Geometry check sheet. Reference: the model listing, model coordinates, mm. Face numbers are marked on the shaded views. A direction names the side the tool comes from. Give positions to 0.01 mm unless a question says otherwise; leave off trailing zeros. Loops run counter-clockwise (first coordinate to the right, second up) from the corner with the lowest first, then second, coordinate; pieces in that order, holes last.
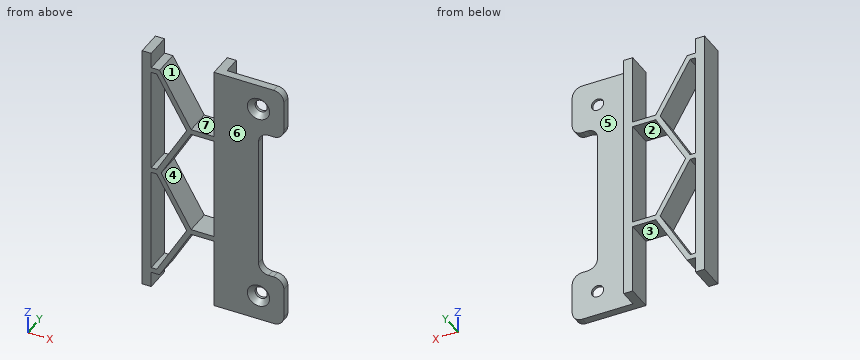
```python
from build123d import *

# Parameters (mm, degrees)
BOSS_EXTRUDE1_DEPTH                            = 5
BOSS_EXTRUDE3_DEPTH                            = 1.5
FILLET1_R                                      = 2
CSK_FOR_M2_FLAT_HEAD_MACHINE_SCREW1_AT_2_COUNT = 2
CSK_FOR_M2_FLAT_HEAD_MACHINE_SCREW1_AT_2_PITCH = 40


with BuildPart() as part:
    # Sketch1 → Boss-Extrude1 (new body)
    with BuildSketch(Plane(origin=(0, 0, 0), x_dir=(1, 0, 0), z_dir=(0, 1, 0))):
        Polygon((-14.18, 46.928571429), (-14.18, 50), (-15.96, 50), (-15.96, 0), (-14.18, 0), (-14.18, 3.071428571), (-12.513875906, 3.071428571), (-6.313875906, 13.785714286), (-1.78, 13.785714286), (-1.78, 0), (0, 0), (0, 50), (-1.78, 50), (-1.78, 36.214285714), (-6.313875906, 36.214285714), (-12.513875906, 46.928571429), align=None)
        Polygon((-14.18, 4.071428571), (-14.18, 24.5), (-13.090568539, 24.5), (-7.179901872, 14.285714286), (-13.090568539, 4.071428571), align=None, mode=Mode.SUBTRACT)
        Polygon((-13.090568539, 45.928571429), (-7.179901872, 35.714285714), (-13.090568539, 25.5), (-14.18, 25.5), (-14.18, 45.928571429), align=None, mode=Mode.SUBTRACT)
        Polygon((-6.313875906, 14.785714286), (-12.224542572, 25), (-6.313875906, 35.214285714), (-1.78, 35.214285714), (-1.78, 14.785714286), align=None, mode=Mode.SUBTRACT)
    extrude(amount=BOSS_EXTRUDE1_DEPTH)

    # Sketch5 → Boss-Extrude3 (add)
    with BuildSketch(Plane.XZ):
        Polygon((12, -40), (12, -50), (0, -50), (0, 0), (12, 0), (12, -10), (7, -10), (7, -40), align=None)
    extrude(amount=-BOSS_EXTRUDE3_DEPTH)

    # Fillet1
    fillet1_edges = [part.edges().sort_by_distance(p)[0] for p in [
        (12, 0.75, 0),
        (12, 0.75, -10),
        (7, 0.75, -10),
        (7, 0.75, -40),
        (12, 0.75, -40),
        (12, 0.75, -50),
    ]]
    fillet(fillet1_edges, radius=FILLET1_R)

    # Sketch6 → CSK for M2 Flat Head Machine Screw1 (revolve, cut)
    with BuildSketch(Plane(origin=(7, 0, -5), x_dir=(0, 0, -1), z_dir=(1, 0, 0))):
        Polygon((0, 0), (0, 1.5), (1.2, 1.5), (1.2, 1), (2.2, 0), align=None)
    csk_for_m2_flat_head_machine_screw1 = revolve(axis=Axis((7, -6.35, -5), (0, 1, 0)), mode=Mode.SUBTRACT)

    # CSK for M2 Flat Head Machine Screw1 at 2: CSK for M2 Flat Head Machine Screw1 ×2
    with Locations(*[(0, 0, -i * CSK_FOR_M2_FLAT_HEAD_MACHINE_SCREW1_AT_2_PITCH) for i in range(1, CSK_FOR_M2_FLAT_HEAD_MACHINE_SCREW1_AT_2_COUNT)]):
        add(csk_for_m2_flat_head_machine_screw1, mode=Mode.SUBTRACT)


solid = part.part
```
1) Sectioned sample at B-B on z = -41.5. Enter the section's corners in (x, y), plus the area to 3 significant figures.
2) Sectioned sample at A-A on x = -5. Enter the section's corners in (y, z), plus the area to 3 significant figures.
3) Sectioned sample at D-D on z = -5. Enter the section's corners in (x, y), plus the area to 3 significant figures.
4) Scan lines: line 1 along X through (y, z) = (1.45, -45); line 2 along X through (y, z) = (2.7, -36.5); line 3 along X through (y, z) = (3.15, -38.5). Record each from-to range of solid material in increasing order.
5) Mould release check, pull along Z, two halves, no side actions. Record for the marked faces 1, 2 and 3: +Z half, -Z half, draft (parallel to the pull), parting line (faces both ways), or undercut.
6) Sectioned sample at C-C on x = -8.25. Enter the section's corners in (y, z), plus the area to 3 significant figures.
7) Depth check by flat-ended pin: P1, Ø1.6, axis at y = 0.5, z = -30.5, coming from the +X side; P2, Ø1.5, axis at y = 3.5, z = -19, coming from the +X side; P3, Ø10, axis at x = 8.5, z = -14, coming from the +Y side. Enter the tip coordinate at first touch or a pass-through.
8) Tool access check on the marked faces 4, 5, 6 and 7. Record the directions out of +Z, -Z, +X, -X, +Y, -Y that give a thin tool (end or side, any length) a straight path to the whole face; none if there is none.
Determined:
1. outline: (-15.96, 0) - (-14.18, 0) - (-14.18, 5) - (-15.96, 5) - close; (-10.53, 0) - (-9.37, 0) - (-9.37, 5) - (-10.53, 5) - close; (-1.78, 0) - (11.94, 0) - (11.94, 1.5) - (0, 1.5) - (0, 5) - (-1.78, 5) - close
1. area: 41.5 mm2
2. outline: (0, -36.21) - (5, -36.21) - (5, -35.21) - (0, -35.21) - close; (0, -14.79) - (5, -14.79) - (5, -13.79) - (0, -13.79) - close
2. area: 10.0 mm2
3. outline: (-15.96, 0) - (-14.18, 0) - (-14.18, 5) - (-15.96, 5) - close; (-12.55, 0) - (-11.4, 0) - (-11.4, 5) - (-12.55, 5) - close; (-1.78, 0) - (4.8, 0) - (5.8, 1) - (5.8, 1.5) - (0, 1.5) - (0, 5) - (-1.78, 5) - close; (8.2, 1) - (9.2, 0) - (12, 0) - (12, 1.5) - (8.2, 1.5) - close
3. area: 37.0 mm2
4. line 1: x = -15.96 to -14.18, -12.55 to -11.4, -1.78 to 5.8, 8.2 to 12
4. line 2: x = -15.96 to -14.18, -7.63 to -6.48, -1.78 to 0
4. line 3: x = -15.96 to -14.18, -8.79 to -7.64, -1.78 to 0
5. face 1: +Z half
5. face 2: undercut
5. face 3: -Z half
6. outline: (0, -39.56) - (5, -39.56) - (5, -37.56) - (0, -37.56) - close; (0, -33.87) - (5, -33.87) - (5, -31.87) - (0, -31.87) - close; (0, -18.13) - (5, -18.13) - (5, -16.13) - (0, -16.13) - close; (0, -12.44) - (5, -12.44) - (5, -10.44) - (0, -10.44) - close
6. area: 39.9 mm2
7. P1: stops at x = 7
7. P2: stops at x = 0
7. P3: stops at y = 1.5
8. face 4: +Y, -Y
8. face 5: +Z, -Z, +X, +Y
8. face 6: +Z, -Z, +X, -X, -Y
8. face 7: +Z, +Y, -Y
